Could you check a few things on this model? Use its own coordinates, in mm. Face numbers are marked on the shaded views. A direction names the side the tool comes from. Give positions to 0.01 mm unless a question says otherwise; leave off trailing zeros. Loops run counter-clockwise (first coordinate to the right, second up) from the corner with the lowest first, then second, coordinate; pieces in that order, holes last. Notation, with made-up numbers: (24.25, 30) -> (64.25, 30) arc R12 cw to (64.25, 52) -> close; hole circle Ø6 at (68, 78). An arc over 180 degrees is marked (long way). Write item = value, one per line. Start each with the question number.
1) I want a section at B-B (y = 0). List the corners of the cut face in (x, z) for me (3 decimals), and give its area (3 significant figures).
2) On a 3-axis mill with a long thin cutter (end or side, diameter ignored), from which of +Z, -Z, +X, -X, +Y, -Y can I reach the whole of each face in a straight line? I mean the marked faces 1 and 2. Say none if no direction works.
3) I'm going to push a flat-ended pin straight in: pin 1 Ø2 at (x, y) = (-47, -26.5) entering from +Z. Where does the tip first touch, or does it pass through?
4) I need wall thicknesses on probe 1 along X at (y, z) = (-34.5, 55.5); probe 2 along Y at (x, z) = (0, 3) (3 decimals); probe 3 along Z at (x, y) = (-40, 16). Which ranges of each line are inside material? Lowest first, please. Write a range as from..to.
5) If we mould it in two halves opening along X, with no side actions, what happens to the marked faces 3, 4 and 5? For each: +X half, -X half, draft (parallel to the pull), parting line (faces both ways), or undercut.
6) I want a section at D-D (z = 42.5). List the corners of the cut face in (x, y) for me.
7) I want a section at A-A (x = 0). List the corners of the cut face in (y, z) for me (3 decimals), and give its area (3 significant figures).
8) I want a section at C-C (z = 31). List the corners of the cut face in (x, y) for me.
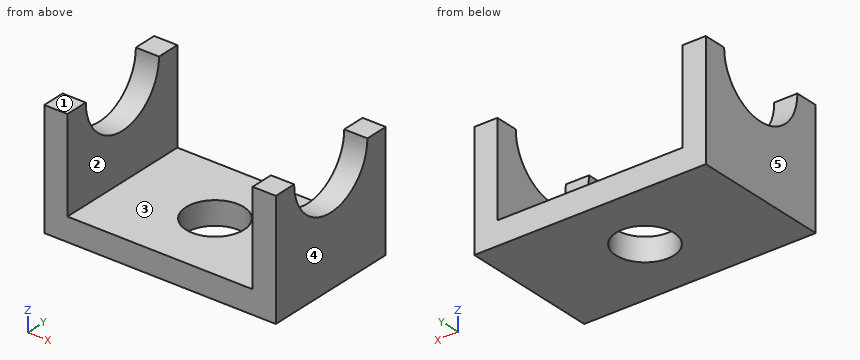
from build123d import *

# Parameters (mm, degrees)
F0_R     = 15.875
F0_W     = 12.7
F0_H     = 76.2
F1_DEPTH = 12.7
F2_DEPTH = 63.5
F4_DEPTH = 127.001


with BuildPart() as f1:
    # F0 (on Top) → F1 (new body)
    with BuildSketch(Plane.XY):
        Polygon((50.8, -38.1), (50.8, 38.1), (-50.8, 38.1), (-50.8, -38.1), (0, -38.1), align=None)
        Circle(F0_R, mode=Mode.SUBTRACT)
        with Locations((-57.15, 0)):
            Rectangle(F0_W, F0_H)
        Polygon((63.5, 0), (63.5, 38.1), (50.8, 38.1), (50.8, -38.1), (63.5, -38.1), align=None)
    extrude(amount=F1_DEPTH)

    # F0 (on Top) → F2 (join)
    with BuildSketch(Plane.XY):
        with Locations((-57.15, 0)):
            Rectangle(F0_W, F0_H)
        Polygon((63.5, 0), (63.5, 38.1), (50.8, 38.1), (50.8, -38.1), (63.5, -38.1), align=None)
    extrude(amount=F2_DEPTH)

    # F3 (on face) → F4 (cut, through all)
    with BuildSketch(Plane.YZ.offset(63.5)):
        with BuildLine():
            ThreePointArc((-25.4, 63.5), (0, 38.1), (25.4, 63.5))
            Line((25.4, 63.5), (-25.4, 63.5))
        make_face()
    extrude(amount=-F4_DEPTH, mode=Mode.SUBTRACT)


solid = f1.part
Answer list:
q1.outline = (-63.5, 0) -> (-15.875, 0) -> (-15.875, 12.7) -> (-50.8, 12.7) -> (-50.8, 38.1) -> (-63.5, 38.1) -> close; (15.875, 0) -> (63.5, 0) -> (63.5, 38.1) -> (50.8, 38.1) -> (50.8, 12.7) -> (15.875, 12.7) -> close
q1.area = 1,850 mm^2
q2.face_1 = +Z, +X, -X, +Y, -Y
q2.face_2 = +Z, +Y, -Y
q3.pin_1 = 12.7
q4.probe_1 = -63.5..-50.8, 50.8..63.5
q4.probe_2 = -38.1..-15.875, 15.875..38.1
q4.probe_3 = 0..12.7
q5.face_3 = undercut
q5.face_4 = +X half
q5.face_5 = -X half
q6.outline = (-63.5, -38.1) -> (-50.8, -38.1) -> (-50.8, -14.29) -> (-63.5, -14.29) -> close; (-63.5, 14.29) -> (-50.8, 14.29) -> (-50.8, 38.1) -> (-63.5, 38.1) -> close; (50.8, -38.1) -> (63.5, -38.1) -> (63.5, -14.29) -> (50.8, -14.29) -> close; (50.8, 14.29) -> (63.5, 14.29) -> (63.5, 38.1) -> (50.8, 38.1) -> close
q7.outline = (-38.1, 0) -> (-15.875, 0) -> (-15.875, 12.7) -> (-38.1, 12.7) -> close; (15.875, 0) -> (38.1, 0) -> (38.1, 12.7) -> (15.875, 12.7) -> close
q7.area = 565 mm^2
q8.outline = (-63.5, -38.1) -> (-50.8, -38.1) -> (-50.8, 38.1) -> (-63.5, 38.1) -> close; (50.8, -38.1) -> (63.5, -38.1) -> (63.5, 38.1) -> (50.8, 38.1) -> close
